The listing builds one solid part. Answer for the finished solid, in the listing's coordinates (mm). Face numbers are marked on the shaded views. A direction names the side the tool comes from. Give positions to 0.01 mm unless a question says otherwise; leave off trailing zeros. Loops run counter-clockwise (first coordinate to the right, second up) from the corner with the lowest first, then second, coordinate; pieces in that order, holes last. Notation, with made-up numbers: (-36.5, 70.25) - (14.5, 70.25) arc R10 ccw to (14.5, 75.25) - close; hole circle Ø7 at (70, -35). An arc over 180 degrees is marked (long way). Answer as CSV lines item,"result". Start each with the question number.
1) Flat-ended cylindrical pins translate along their axes: pin 1 (4 mm diameter, centred on x = 3, z = 2, fed in from +Y); pin 2 (5 mm diameter, centred on x = 13.5, y = 6, fed in from +Z); pin 3 (3 mm diameter, centred on x = 8.5, z = 3.5, fed in from +Y). Find the tip coordinate at first contact, or state that the pin passes through.
2) Find the intervals of material crossed by line 1 along X through (y, z) = (7.5, 0.5); line 2 along Y through (x, z) = (19, 1.25); line 3 along Z through (x, y) = (12.25, 3), in increasing order.
3) A cutting plane is placed at A-A (y = 28.5). Determine the outline of the cut face in (x, z), and give its area (3 significant figures).
4) A cutting plane is placed at B-B (z = 0.5). Determine the outline of the cut face in (x, y), and give its area (4 significant figures).
5) A cutting plane is placed at C-C (x = 14.5). Determine the outline of the cut face in (y, z).
6) For a pull along X with two mould halves and no side action, classify the marked faces 1, 2, 3 and 4 as pulls with the +X half, pulls with the -X half, needs draft (parallel to the pull), parting line crosses it, or undercut.
7) For the marked faces 5 and 6, determine the directions among +Z, -Z, +X, -X, +Y, -Y from which every point of the face is accessible in a straight line to the end or side of a thin tool.
Autodesk Inventor part; units mm, degrees
sketch "Skizze1" plane through (0, 0, 0) normal (0, 0, 1) x (1, 0, 0)
  line L0 (0, 0) -> (23, 0)
  line L1 (23, 0) -> (23, 30.5)
  line L2 (23, 30.5) -> (0, 30.5)
  line L3 (0, 30.5) -> (0, 0)
  dimension "d0" = 23
  dimension "d1" = 30.5
extrude "Extrusion1" add sketch "Skizze1" along normal mid plane 10
sketch "Skizze2" plane through (0, 0, 5) normal (0, 0, 1) x (1, 0, 0)
  line L0 (2.5, 28) -> (20.5, 28)
  line L1 (20.5, 28) -> (20.5, 2.5)
  line L2 (20.5, 2.5) -> (2.5, 2.5)
  line L3 (2.5, 2.5) -> (2.5, 28)
  point P0 (0, 0)
  dimension "d4" = 18
  dimension "d5" = 25.5
extrude "Extrusion2" cut sketch "Skizze2" against normal blind 5
sketch "Skizze3" plane through (0, 30.5, 5) normal (0, 1, 0) x (1, 0, 0)
  line L0 (23, 0) -> (0, 0)
  line L1 (2.5, 5) -> (20.5, 5)
  line L2 (2.5, 0) -> (20.5, 0)
  line L3 (20.5, 0) -> (20.5, 5)
  line L4 (20.5, 5) -> (2.5, 5)
  line L5 (2.5, 5) -> (2.5, 0)
  point P0 (0, 5)
  dimension "d8" = 18
  dimension "d9" = 5
extrude "Extrusion3" cut sketch "Skizze3" against normal blind 5
properties part number "espverkleidung"
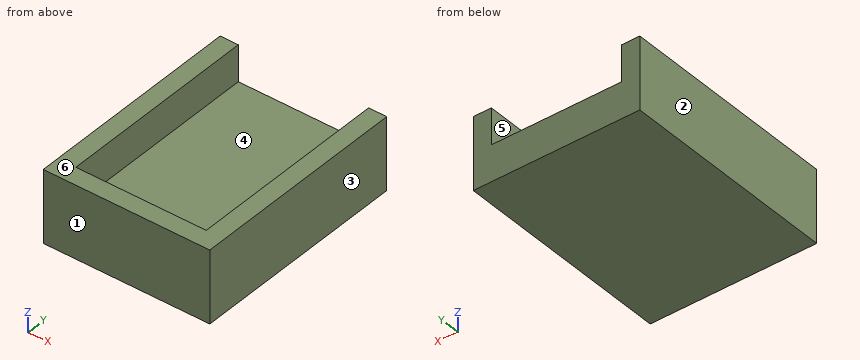
Ans:
1,pin 1,"y = 30.5"
1,pin 2,"z = 0"
1,pin 3,"y = 2.5"
2,line 1,"0 to 2.5, 20.5 to 23"
2,line 2,"0 to 2.5"
2,line 3,"-5 to 0"
3,outline,"(0, -5) - (23, -5) - (23, 5) - (20.5, 5) - (20.5, 0) - (2.5, 0) - (2.5, 5) - (0, 5) - close"
3,area,"140 mm2"
4,outline,"(0, 0) - (23, 0) - (23, 30.5) - (20.5, 30.5) - (20.5, 2.5) - (2.5, 2.5) - (2.5, 30.5) - (0, 30.5) - close"
4,area,"197.5 mm2"
5,outline,"(0, -5) - (30.5, -5) - (30.5, 0) - (2.5, 0) - (2.5, 5) - (0, 5) - close"
6,face 1,"needs draft"
6,face 2,"pulls with the -X half"
6,face 3,"pulls with the +X half"
6,face 4,"undercut"
7,face 5,"+Z, +Y"
7,face 6,"+Z, +X, -X, +Y, -Y"
